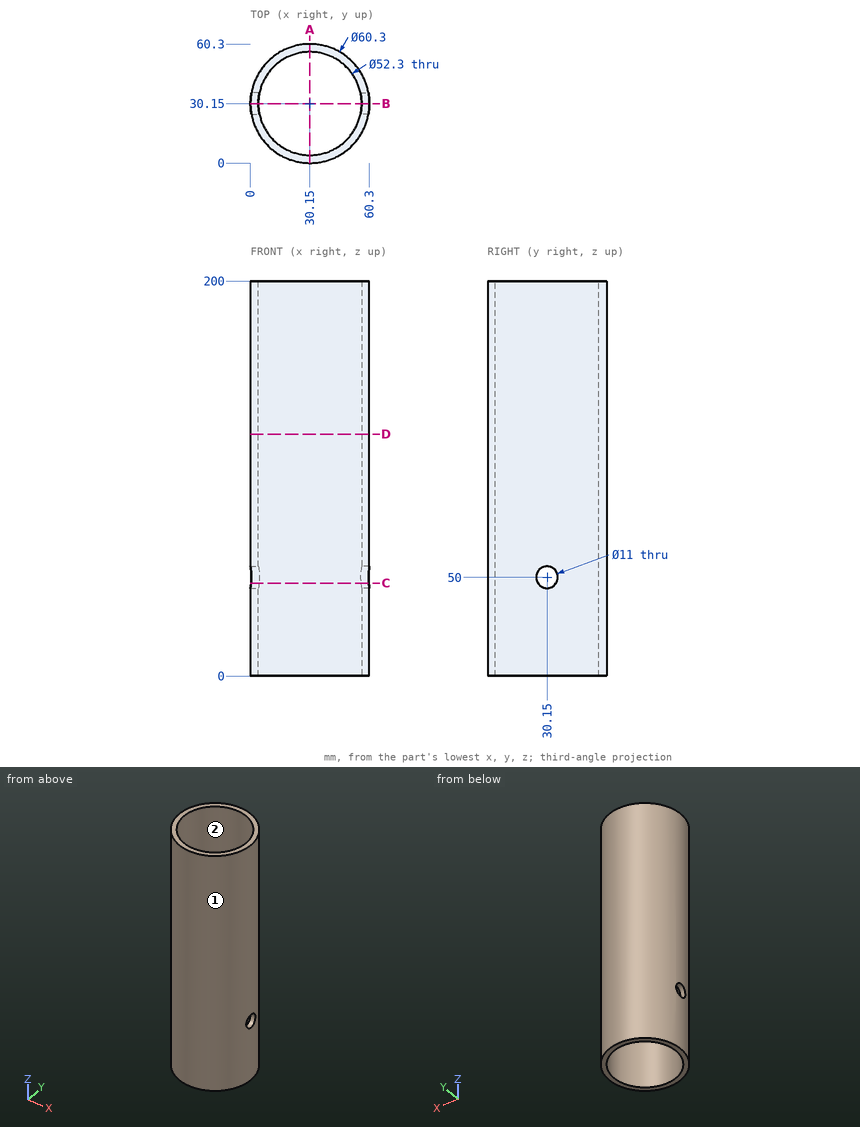
Here's the drawing with two shaded views (mm, measured from the low corner). I have some questions. Give positions to 0.01 mm unless a question says otherwise; leave off trailing zeros. Order: outer loops, then holes, each group sorted by start corner. A loop starts at its lowest first (then second) coordinate and runs counter-clockwise, first axis right, second up.
Q1. Suppose I cut it at A-A, the plane x = 30.15. Write out the boundary of the cut face in (y, z), and give its area (3 significant figures).
Q2. I'm going to push flat-ended pins straight in: P1, Ø17.5, axis at y = 30.15, z = 50, coming from the +X side; P2, Ø2, axis at x = 15.5, z = 132, coming from the +Y side; P3, Ø5, axis at x = 39, y = 9.5, coming from the -Z side; P4, Ø4, axis at x = 36, z = 177, coming from the -Y side. Where does each tip first touch, or does it pass through?
Q3. Suppose I cut it at C-C, the plane z = 47. Write out the boundary of the cut face in (x, y).
Q4. If I drill on line 1 along X through (y, z) = (30, 80); line 2 along Z through (x, y) = (58, 30), over which ranges is the centre line in solid material (lowest first)?
Q5. Suppose I cut it at D-D, the plane z = 122.5. Write out the boundary of the cut face in (x, y).
Q6. Suppose I cut it at B-B, the plane y = 30.15. Write out the boundary of the cut face in (x, z).
Q7. We'd pull the mould along X, two halves only. Please class the marked faces 1 and 2: +X half, -X half, draft (parallel to the pull), parting line (faces both ways), or undercut.
Solution:
1. outline: (0, 0) - (4, 0) - (4, 200) - (0, 200) - close; (56.3, 0) - (60.3, 0) - (60.3, 200) - (56.3, 200) - close
1. area: 1,600 mm2
2. P1: stops at x = 60.3
2. P2: stops at y = 57.03
2. P3: passes through
2. P4: stops at y = 0.25
3. outline: (0.35, 25.54) arc R30.15 ccw to (59.95, 25.54) - (55.89, 25.54) arc R26.15 cw to (4.41, 25.54) - close; (0.35, 34.76) - (4.41, 34.76) arc R26.15 cw to (55.89, 34.76) - (59.95, 34.76) arc R30.15 ccw to start
4. line 1: x = 0 to 4, 56.3 to 60.3
4. line 2: z = 0 to 44.5, 55.5 to 200
5. outline: circle Ø60.3 at (30.15, 30.15); hole circle Ø52.3 at (30.15, 30.15)
6. outline: (0, 0) - (4, 0) - (4, 44.5) - (0, 44.5) - close; (0, 55.5) - (4, 55.5) - (4, 200) - (0, 200) - close; (56.3, 0) - (60.3, 0) - (60.3, 44.5) - (56.3, 44.5) - close; (56.3, 55.5) - (60.3, 55.5) - (60.3, 200) - (56.3, 200) - close
7. face 1: parting line
7. face 2: undercut
